```python
from build123d import *

# Parameters (mm, degrees)
SKETCH1_W           = 13
SKETCH1_H           = 33.5
BOSS_EXTRUDE1_DEPTH = 16.7
SKETCH2_R           = 6
BOSS_EXTRUDE2_DEPTH = 9
SKETCH4_R           = 5
CUT_EXTRUDE1_DEPTH  = 4
SKETCH5_R           = 3
BOSS_EXTRUDE3_DEPTH = 21.5
REVOLVE2_ANGLE      = 180
FILLET1_R           = 2


with BuildPart() as part:
    # Sketch1 → Boss-Extrude1 (new body)
    with BuildSketch(Plane(origin=(0, 0, 0), x_dir=(1, 0, 0), z_dir=(0, 1, 0))):
        Rectangle(SKETCH1_W, SKETCH1_H)
    extrude(amount=BOSS_EXTRUDE1_DEPTH)

    # Sketch2 → Boss-Extrude2 (add)
    with BuildSketch(Plane(origin=(0, 16.7, 0), x_dir=(1, 0, 0), z_dir=(0, 1, 0))):
        with Locations(Location((0, 0, 0), (0, 0, 270))):  # turned: the seam where the file's is
            Circle(SKETCH2_R)
    extrude(amount=BOSS_EXTRUDE2_DEPTH)

    # Sketch4 → Cut-Extrude1 (cut)
    with BuildSketch(Plane(origin=(0, 25.7, 0), x_dir=(1, 0, 0), z_dir=(0, 1, 0))):
        with Locations(Location((0, 0, 0), (0, 0, 270))):  # turned: the seam where the file's is
            Circle(SKETCH4_R)
    extrude(amount=-CUT_EXTRUDE1_DEPTH, mode=Mode.SUBTRACT)

    # Sketch5 → Boss-Extrude3 (add)
    with BuildSketch(Plane(origin=(0, 21.7, 0), x_dir=(1, 0, 0), z_dir=(0, 1, 0))):
        with Locations(Location((0, 0, 0), (0, 0, 270))):  # turned: the seam where the file's is
            Circle(SKETCH5_R)
    extrude(amount=BOSS_EXTRUDE3_DEPTH)

    # Sketch3 → Revolve2 (revolve)
    with BuildSketch(Plane(origin=(0, 21.7, 0), x_dir=(1, 0, 0), z_dir=(0, 1, 0))):
        with BuildLine():
            Line((0, -5), (0, 5))
            ThreePointArc((0, 5), (-5, 0), (0, -5))
        make_face()
    revolve(axis=Axis((0, 21.7, 6), (0, 0, -1)), revolution_arc=REVOLVE2_ANGLE)

    # Fillet1
    fillet1_edges = [part.edges().sort_by_distance(p)[0] for p in [
        (0, 43.2, -3),
    ]]
    fillet(fillet1_edges, radius=FILLET1_R)


solid = part.part
```
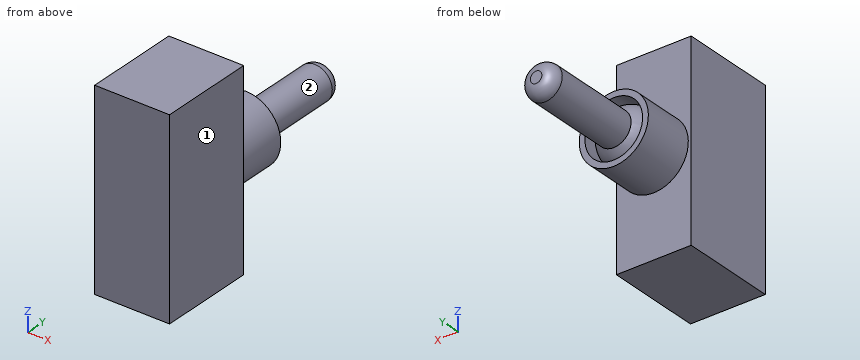
Input: part model. Units: mm. Frame: model coordinates. Face numbers are marked on the shaded views. A direction names the side the tool comes from. Give positions to 0.01 mm unless a question says otherwise; leave off trailing zeros. Loops run counter-clockwise (first coordinate to the right, second up) from the corner with the lowest first, then second, coordinate; pieces in that order, holes last. Notation, with made-up numbers: (-17, 16) -> (-3, 16) arc R27 ccw to (-3, 48) -> close; hole circle Ø2 at (59, 28.5). An arc over 180 degrees is marked (long way). Use a Markdown table: item, result.
Q1. Section query D-D, the plane z = 11. Return the cut outline in (x, y), plus the area to 3 significant figures.
Entries:
| item | result |
|---|---|
| outline | (-6.5, 0) -> (6.5, 0) -> (6.5, 16.7) -> (-6.5, 16.7) -> close |
| area | 217 mm² |
Q2. Access query for the marked faces 1 and 2. Directions: +Z, -Z, +X, -X, +Y, -Y. A direction counts if a zero-diameter tool reaches every point of the face in a straight line with its end or side. Return the directions, or none.
Entries:
| item | result |
|---|---|
| face 1 | +Z, -Z, +X, +Y, -Y |
| face 2 | +Y |
Q3. Ray query, probe 1 along X at (y, z) = (24.85, 0); probe 2 along Y at (x, z) = (-0.75, -5); probe 3 along X at (y, z) = (24, 0). Return the intervals inside material, ascending. Write a range as from..to.
Entries:
| item | result |
|---|---|
| probe 1 | x = -6..-5, -3.88..3.88, 5..6 |
| probe 2 | y = 0..25.7 |
| probe 3 | x = -6..-5, -4.44..4.44, 5..6 |
Q4. Section query A-A, the plane z = 4. Return the cut outline in (x, y).
Entries:
| item | result |
|---|---|
| outline | (-6.5, 0) -> (6.5, 0) -> (6.5, 16.7) -> (4.47, 16.7) -> (4.47, 25.7) -> (3, 25.7) -> (3, 21.7) arc R3 ccw to (-3, 21.7) -> (-3, 25.7) -> (-4.47, 25.7) -> (-4.47, 16.7) -> (-6.5, 16.7) -> close |
Q5. First-contact query: P1, Ø3, axis at y = 21, z = -1.5, coming from the +X side; P2, Ø1, axis at x = -0.5, z = -13, coming from the +Y side; P3, Ø1, axis at x = 2, y = 34.5, coming from the +Z side. Flat tips, straight axial feed; report the tip coordinate or a pass-through.
Entries:
| item | result |
|---|---|
| P1 | stops at x = 6 |
| P2 | stops at y = 16.7 |
| P3 | stops at z = 2.6 |
Q6. Section query B-B, the plane x = -5.5. Return the cut outline in (y, z), plus the area to 3 significant figures.
Entries:
| item | result |
|---|---|
| outline | (0, -16.75) -> (16.7, -16.75) -> (16.7, -2.4) -> (25.7, -2.4) -> (25.7, 2.4) -> (16.7, 2.4) -> (16.7, 16.75) -> (0, 16.75) -> close |
| area | 603 mm² |
Q7. Section query C-C, the plane y = 39. Return the cut outline in (x, z), plus the area to 3 significant figures.
Entries:
| item | result |
|---|---|
| outline | circle Ø6 at (0, 0) |
| area | 28.3 mm² |
